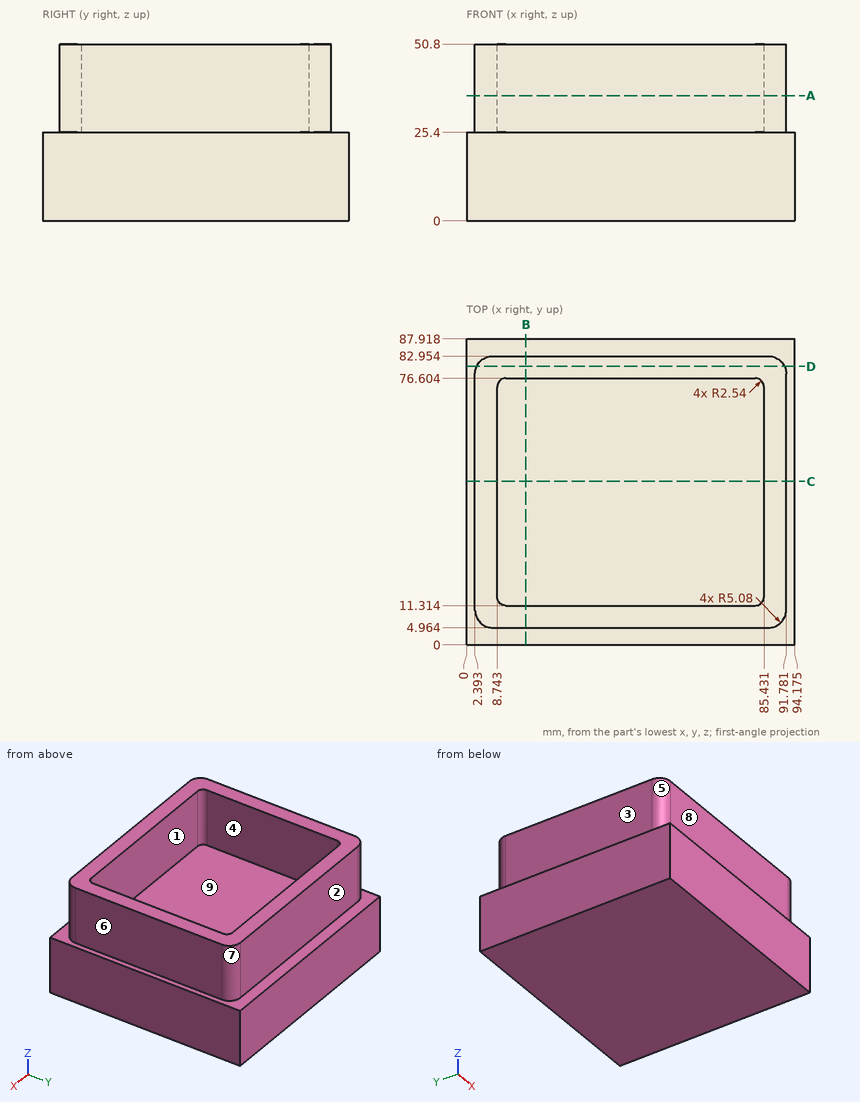
For this review, use the dimensioned drawing (mm, ordinates from the lowest corner) and the shaded views. A direction names the side the tool comes from. Give positions to 0.01 mm unless a question says otherwise; leave off trailing zeros. Order: outer loops, then holes, each group sorted by start corner. A loop starts at its lowest first (then second) coordinate and runs counter-clockwise, first axis right, second up.
1) The part is to be moulded in two halves that separate along X. For the marked faces 1, 2, 3 and 4, say which applies: released by +X, released by -X, zero draft, split by the parting line, or undercut.
2) Take a section at A-A (z = 36). Give the boundary of the cut face in (x, y) (1 decimal).
3) Take a section at B-B (x = 17). Give the boundary of the cut face in (y, z) (1 decimal).
4) Wall thickness on line 1 (Y direction, x = 63, z = 46.5) (1 decimal); line 2 (Z direction, x = 46, y = 62); line 3 (X direction, y = 75, z = 49) (1 decimal): over which ranges is each line inside the solid? List them lowest first.
5) Take a section at C-C (y = 47). Give the boundary of the cut face in (x, z) (1 decimal).
6) For the marked faces 5, 6, 7, 8 and 9, list the 3-axis set-ups (+Z, -Z, +X, -X, +Y, -Y) from which the entire face can be reached by the end or side of a thin tool; tool diameter is ignored.
7) Take a section at D-D (y = 80). Give the boundary of the cut face in (x, z) (1 decimal).
8) Insertion check: pin 1 (8 mm diameter, centred on x = 80.5, z = 32.5, fed in from -Y); pin 2 (12.5 mm diameter, centred on x = 62, z = 37, fed in from +Y); pin 3 (7.5 mm diameter, centred on y = 39, z = 33, fed in from -X). Each pin has a flat end and moves straight along its axis. Give the tip position at first contact, or say it passes through.
Derived:
1. face 1: undercut
1. face 2: zero draft
1. face 3: released by -X
1. face 4: undercut
2. outline: (2.4, 10) arc R5.1 ccw to (7.5, 5) - (86.7, 5) arc R5.1 ccw to (91.8, 10) - (91.8, 77.9) arc R5.1 ccw to (86.7, 83) - (7.5, 83) arc R5.1 ccw to (2.4, 77.9) - close; hole (8.7, 13.9) arc R2.5 ccw to (11.3, 11.3) - (82.9, 11.3) arc R2.5 ccw to (85.4, 13.9) - (85.4, 74.1) arc R2.5 ccw to (82.9, 76.6) - (11.3, 76.6) arc R2.5 ccw to (8.7, 74.1) - close
3. outline: (0, 0) - (87.9, 0) - (87.9, 25.4) - (83, 25.4) - (83, 50.8) - (76.6, 50.8) - (76.6, 25.4) - (11.3, 25.4) - (11.3, 50.8) - (5, 50.8) - (5, 25.4) - (0, 25.4) - close
4. line 1: y = 5 to 11.3, 76.6 to 83
4. line 2: z = 0 to 25.4
4. line 3: x = 2.4 to 8.9, 85.3 to 91.8
5. outline: (0, 0) - (94.2, 0) - (94.2, 25.4) - (91.8, 25.4) - (91.8, 50.8) - (85.4, 50.8) - (85.4, 25.4) - (8.7, 25.4) - (8.7, 50.8) - (2.4, 50.8) - (2.4, 25.4) - (0, 25.4) - close
6. face 5: +Z, -X, -Y
6. face 6: +Z, +X, +Y, -Y
6. face 7: +Z, +X, +Y
6. face 8: +Z, +X, -X, -Y
6. face 9: +Z
7. outline: (0, 0) - (94.2, 0) - (94.2, 25.4) - (91.3, 25.4) - (91.3, 50.8) - (2.9, 50.8) - (2.9, 25.4) - (0, 25.4) - close
8. pin 1: stops at y = 4.96
8. pin 2: stops at y = 82.95
8. pin 3: stops at x = 2.39
